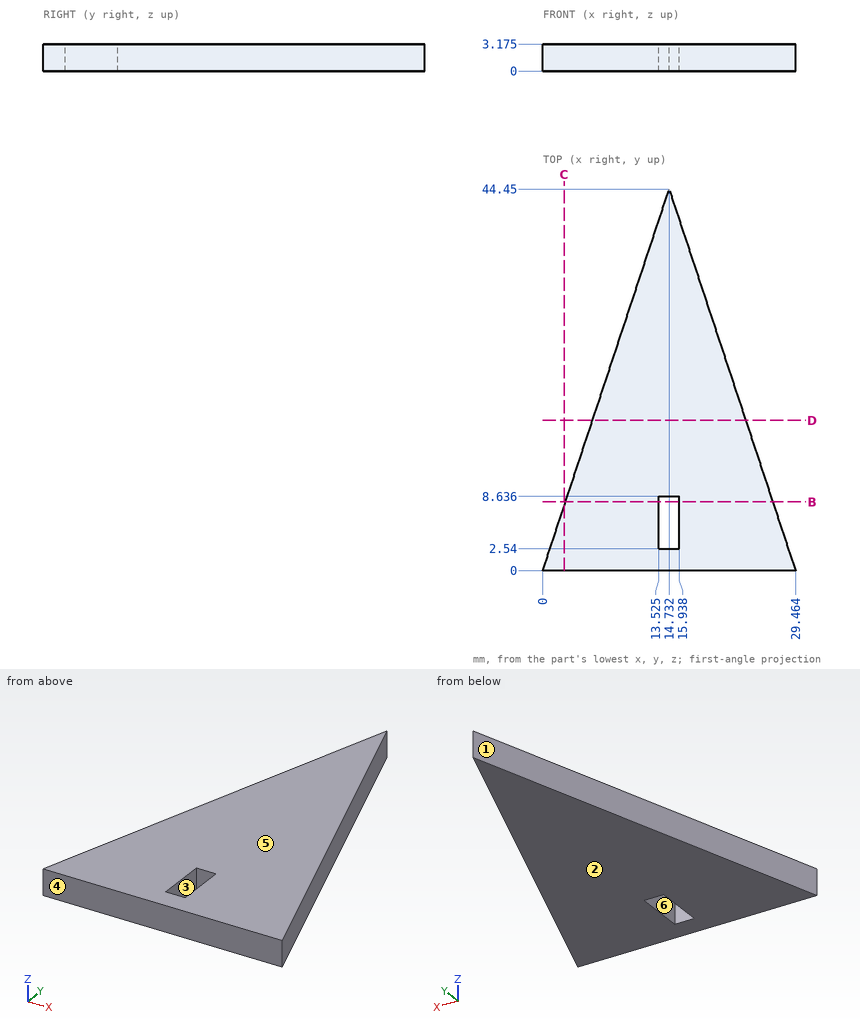
Geometry: see drawing. Coordinates: mm, zero at the bounding-box minimum. A direction names the side the tool comes from. Give positions to 0.01 mm unless a question says otherwise; leave off trailing zeros. Order: outer loops, then holes, each group sorted by start corner. A loop starts at its lowest first (then second) coordinate and runs counter-clockwise, first axis right, second up.
1. Cut plane C-C (x = 2.5). Return loops of the section in (y, z) (1 decimal).
Computed:
outline: (0, 0) - (7.5, 0) - (7.5, 3.2) - (0, 3.2) - close
2. Cut plane B-B (y = 8). Return loops of the section in (x, z) (1 decimal).
Computed:
outline: (2.7, 0) - (13.5, 0) - (13.5, 3.2) - (2.7, 3.2) - close; (15.9, 0) - (26.8, 0) - (26.8, 3.2) - (15.9, 3.2) - close
3. Pin query (flat end, axial travel): pin 1 Ø1.6 at (y, z) = (5, 2) entering from -X; pin 2 Ø10 at (x, y) = (4, 39) entering from -Z. Return the tip coordinate at first contact, or that it passes through.
Computed:
pin 1: stops at x = 1.39
pin 2: passes through
4. Draft query along Y for the marked faces 1, 2, 3 and 4. Return one class per face: released by +Y, released by -Y, zero draft, split by the parting line, or undercut.
Computed:
face 1: released by +Y
face 2: zero draft
face 3: undercut
face 4: released by -Y
5. Cut plane D-D (y = 17.5). Return loops of the section in (x, z) (1 decimal).
Computed:
outline: (5.8, 0) - (23.7, 0) - (23.7, 3.2) - (5.8, 3.2) - close
6. Set-up query: the marked faces 5 and 6. Return all of +Z, -Z, +X, -X, +Y, -Y with unobstructed straight access to the full face (end or side cutting, diameter ignored); none if empty.
Computed:
face 5: +Z, +X, -X, +Y, -Y
face 6: +Z, -Z
7. Line query: probe 1 along X at (y, z) = (6, 1.4) (1 decimal); probe 2 along X at (y, z) = (18.5, 0.3); probe 3 along X at (y, z) = (40.5, 1.75). Output: solid intervals per line, ascending.
Computed:
probe 1: x = 2 to 13.5, 15.9 to 27.5
probe 2: x = 6.13 to 23.33
probe 3: x = 13.42 to 16.04
